Study the drawing (mm; zero at the part's minimum x, y, z) and answer. A direction names the side the tool comes from. Give positions to 0.01 mm unless a question says otherwise; leave off trailing zeros. Order: outer loops, then holes, each group sorted by start corner. A loop starts at its lowest first (then second) coordinate and runs counter-clockwise, first axis right, second up. Notation, with made-up numbers: (-39, -3) - (11, -3) arc R23 ccw to (11, 22) - close; hole circle Ø4 at (-5, -9.75). An arc over 180 degrees is marked (long way). Use CSV: the item, a comma, the result in double quotes.
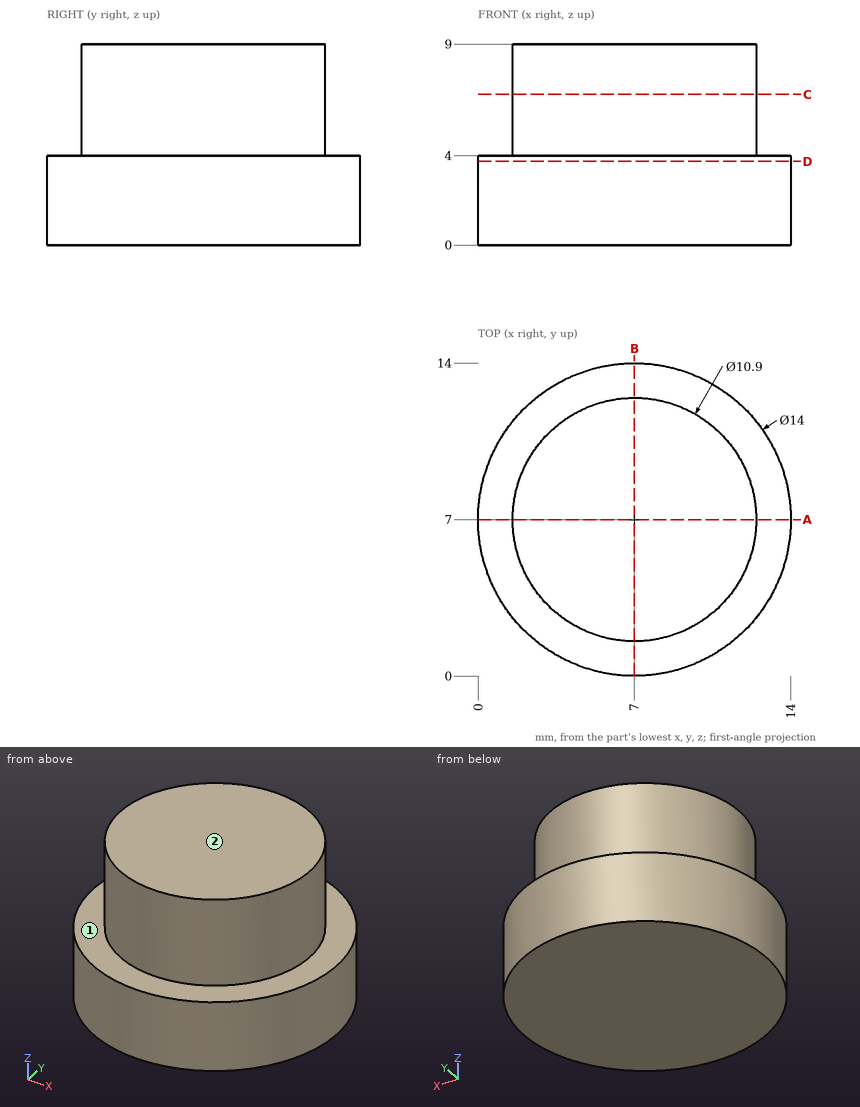
Item 1: The part is cut by section D-D (z = 3.75). Give the vertices of the cut face in (x, y), and give its area (3 significant figures).
Taken from the geometry:
outline,"circle Ø14 at (7, 7)"
area,"154 mm^2"
Item 2: Find the intervals of material crossed by line 1 along Y through (x, z) = (7, 7.5); line 2 along Z through (x, y) = (10.25, 11.75); line 3 along Y through (x, z) = (6.75, 2), in increasing order.
Taken from the geometry:
line 1,"1.55 to 12.45"
line 2,"0 to 4"
line 3,"0 to 14"
Item 3: The part is cut by section A-A (y = 7). Give the vertices of the cut face in (x, z), and give its area (4 significant figures).
Taken from the geometry:
outline,"(0, 0) - (14, 0) - (14, 4) - (12.45, 4) - (12.45, 9) - (1.55, 9) - (1.55, 4) - (0, 4) - close"
area,"110.5 mm^2"
Item 4: Each of these flat-tipped pins is pushed along its axis until it touches: pin 1 (1.5 mm diameter, centred on x = 11, y = 12.5, fed in from +Z); pin 2 (2 mm diameter, centred on y = 11.5, z = 5.5, fed in from -X). Where does it stop, or does it pass through?
Taken from the geometry:
pin 1,"z = 4"
pin 2,"x = 2.82"
Item 5: Which of the six approach directions +Z, -Z, +X, -X, +Y, -Y give full straight-line access (tool end or side, diameter ignored) to the marked faces 1 and 2?
Taken from the geometry:
face 1,"+Z"
face 2,"+Z, +X, -X, +Y, -Y"
Item 6: The part is cut by section C-C (z = 6.75). Give the vertices of the cut face in (x, y).
Taken from the geometry:
outline,"circle Ø10.9 at (7, 7)"
